Verification items for the finished model (mm, model axes). Face numbers are marked on the shaded views. A direction names the side the tool comes from. Round coordinates to 2 decimals unless told otherwise and drop trailing zeros. Order: outer loops, then holes, each group sorted by start corner. A loop starts at its lowest first (then second) coordinate and runs counter-clockwise, first axis right, second up. Notation, with made-up numbers: M 71.25,36 L 129.25,36 A29 cw 129.25,69 Z; hole C 0.5,40.5 d10. An arc over 180 degrees is marked long. Use one line per item in the form item = value. Start each with the question number.
Item 1: Tool access check on the marked faces 4, 5 and 6. Record the directions out of +Z, -Z, +X, -X, +Y, -Y that give a thin tool (end or side, any length) a straight path to the whole face; none if there is none.
Item 2: Go/stop test with flat-tipped pins: pin 1 Ø2 at (y, z) = (-18.5, 18) entering from -X; pin 2 Ø5 at (x, z) = (8.5, -9) entering from -Y; pin 3 Ø4 at (x, y) = (7.5, 7) entering from -Z; pin 4 Ø14.5 at (y, z) = (0, 0) entering from -X. Record where each tip stops, or that it passes through.
Item 3: Cross-section at D-D on x = 8. Enter the section's corners in (y, z), then the cut area to 3 significant figures.
Item 4: Release check for a two-part mould opening along Y. For the marked faces 1, 2 and 3 record: +Y half, -Y half, draft (parallel to the pull), parting line (faces both ways), or undercut.
Item 5: Thickness scan on probe 1 along Y at (x, z) = (2.9, 0); probe 2 along Z at (x, y) = (6.5, 13); probe 3 along Y at (x, z) = (5, 6.5). Record the ranges inside material, lowest first. Write a range as [from, to].
Item 6: Cross-section at B-B on x = 2.25. Enter the section's corners in (y, z), then the cut area to 3 significant figures.
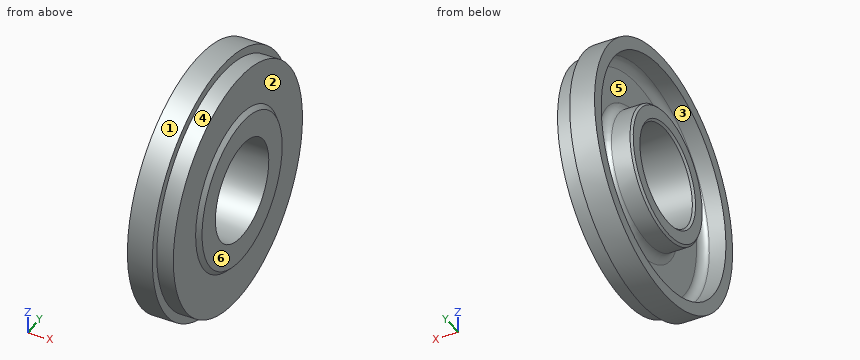
from build123d import *

# Parameters (mm, degrees)
CHANFREIN1_SIZE = 0.5


with BuildPart() as part:
    # Esquisse1 → Base-Révolution (revolve)
    with BuildSketch(Plane.XY, mode=Mode.PRIVATE) as base_r_volution_sk:
        with BuildLine():
            Line((0, 12), (0, 16))
            Line((0, 16), (5, 16))
            ThreePointArc((5, 16), (6.414213562, 16.585786438), (7, 18))
            Line((7, 18), (7, 26))
            ThreePointArc((7, 26), (6.414213562, 27.414213562), (5, 28))
            Line((5, 28), (1, 28))
            Line((1, 28), (1, 31))
            Line((1, 31), (7, 31))
            Line((7, 31), (7, 29))
            Line((7, 29), (11, 29))
            Line((11, 29), (11, 19))
            Line((11, 19), (12, 18))
            Line((12, 18), (12, 12))
            Line((12, 12), (0, 12))
        make_face()
    revolve(base_r_volution_sk.sketch.rotate(Axis((-8, 0, 0), (1, 0, 0)), 90), axis=Axis((-8, 0, 0), (1, 0, 0)))

    # Chanfrein1
    chanfrein1_edges = [part.edges().sort_by_distance(p)[0] for p in [
        (0, 0, -12),
        (0, 0, -16),
    ]]
    chamfer(chanfrein1_edges, length=CHANFREIN1_SIZE)


solid = part.part
Output values:
q1.face_4 = +X
q1.face_5 = -X
q1.face_6 = +Z, -Z, +X, +Y, -Y
q2.pin_1 = 6.83
q2.pin_2 = -30.2
q2.pin_3 = -30.58
q2.pin_4 = through
q3.outline = C 0,0 d58; hole C 0,0 d24
q3.area = 2,190 mm2
q4.face_1 = parting line
q4.face_2 = draft
q4.face_3 = undercut
q5.probe_1 = [-31, -28], [-16, -12], [12, 16], [28, 31]
q5.probe_2 = [-28.14, -24.03], [-10.45, 10.45], [24.03, 28.14]
q5.probe_3 = [-30.31, -27.24], [-14.62, -10.09], [10.09, 14.62], [27.24, 30.31]
q6.outline = C 0,0 d62; C 0,0 d32; hole C 0,0 d56; hole C 0,0 d24
q6.area = 908 mm2
